Autodesk Inventor part; units mm, degrees
ref_plane "YZ Plane" through (0, 0, 0) normal (1, 0, 0) x (0, 1, 0)
ref_plane "XZ Plane" through (0, 0, 0) normal (0, 1, 0) x (-1, 0, 0)
ref_plane "XY Plane" through (0, 0, 0) normal (0, 0, 1) x (1, 0, 0)
sketch "Sketch1" plane through (0, 0, 0) normal (0, 0, 1) x (1, 0, 0)
  line L0 (-15.875, -28.575) -> (25.4, -28.575)
  line L1 (25.4, 28.575) -> (-15.875, 28.575)
  line L2 (-28.575, 15.875) -> (-28.575, -15.875)
  line L3 (-28.575, -28.575) -> (28.575, 28.575) construction
  line L4 (28.575, -28.575) -> (-28.575, 28.575) construction
  arc A0 (-15.875, 28.575) -> (-28.575, 15.875) centre (-15.875, 15.875) ccw
  arc A1 (-28.575, -15.875) -> (-15.875, -28.575) centre (-15.875, -15.875) ccw
  arc A2 (28.575, 25.4) -> (25.4, 28.575) centre (25.4, 25.4) ccw
  arc A3 (25.4, -28.575) -> (28.575, -25.4) centre (25.4, -25.4) ccw
  arc A4 (17.9256, 1.27) -> (17.9256, -1.27) centre (0, 0) ccw
  line L5 (18.2118, 5.08) -> (18.2118, -5.08) construction
  line L6 (17.9256, 1.27) -> (28.575, 1.27)
  line L7 (17.9256, -1.27) -> (28.575, -1.27)
  line L8 (28.575, -25.4) -> (28.575, -1.27)
  line L9 (28.575, 1.27) -> (28.575, 25.4)
  point P0 (23.2503, 1.27)
  point P1 (23.2503, -1.27)
  dimension "d0" = 57.15
  dimension "d1" = 57.15
  dimension "d2" = 12.7
  dimension "d3" = 3.175
  dimension "d5" = 10.16
  dimension "d8" = 28.575
  dimension "d11" = 57.15
  dimension "d14" = 2.54
  dimension "d23" = 35.941
extrude "Extrusion1" add sketch "Sketch1" along normal blind 17.78
sketch "Sketch2" plane through (17.9256, -1.27, 0) normal (0, 1, 0) x (1, 0, 0)
  line L0 (0, 0) -> (10.6494, 0)
  line L1 (0, 0) -> (0, -17.78)
  line L2 (10.6494, -17.78) -> (0, -17.78)
  line L3 (10.6494, 0) -> (10.6494, -17.78)
  circle A0 centre (5.2706, -8.89) radius 1.27
  point P0 (-17.9256, 0)
  dimension "d15" = 2.54
hole "Hole1" at (23.1962, -1.27, 8.89) direction (0, -1, 0) diameter 2.54 end through all
sketch "Sketch3" plane through (-15.875, -28.575, 0) normal (0, -1, 0) x (1, 0, 0)
  circle A0 centre (39.0712, 8.89) radius 1.27
  point P0 (15.875, 0)
  point P1 (38.1, 9.7084)
  point P2 (38.1, 8.0716)
hole "Hole2" at (23.1962, -28.575, 8.89) direction (0, 1, 0) diameter 4.064 end through all counterbore diameter 7.62 counterbore depth 6.35
sketch "Sketch4" plane through (0, 0, 17.78) normal (0, 0, 1) x (1, 0, 0)
  point P0 (0, 0)
sketch "Sketch5" plane through (0, 0, 17.78) normal (0, 0, 1) x (1, 0, 0)
  point P0 (0, 0)
sketch "Sketch6" plane through (0, 0, 17.78) normal (0, 0, 1) x (1, 0, 0)
  line L0 (25.4, 28.575) -> (-15.875, 28.575)
  arc A0 (-15.875, 28.575) -> (-28.575, 15.875) centre (-15.875, 15.875) ccw
  line L1 (-28.575, 15.875) -> (-28.575, -15.875)
  arc A1 (-28.575, -15.875) -> (-15.875, -28.575) centre (-15.875, -15.875) ccw
  line L2 (-15.875, -28.575) -> (25.4, -28.575)
  arc A2 (25.4, -28.575) -> (28.575, -25.4) centre (25.4, -25.4) ccw
  line L3 (28.575, -25.4) -> (28.575, -1.27)
  line L4 (28.575, -1.27) -> (17.9256, -1.27)
  arc A3 (17.9256, 1.27) -> (17.9256, -1.27) centre (0, 0) ccw
  line L5 (17.9256, 1.27) -> (28.575, 1.27)
  line L6 (28.575, 1.27) -> (28.575, 25.4)
  arc A4 (28.575, 25.4) -> (25.4, 28.575) centre (25.4, 25.4) ccw
  circle A5 centre (-19.685, -19.685) radius 1.27
  circle A6 centre (-19.685, 19.685) radius 1.27
  dimension "d31" = 2.54
  dimension "d32" = 3.81
  dimension "d33" = 3.81
  dimension "d34" = 2.54
  dimension "d35" = 3.81
  dimension "d36" = 3.81
extrude "Extrusion2" cut sketch "Sketch6" against normal blind 25.4 contours A5 | A6
properties part number "mOTORHOLDER"
Here's how the part is built. I have some questions about the finished solid (model axes, mm). A direction names the side the tool comes from. Give positions to 0.01 mm unless a question says otherwise; leave off trailing zeros. Order: outer loops, then holes, each group sorted by start corner. A loop starts at its lowest first (then second) coordinate and runs counter-clockwise, first axis right, second up. Notation, with made-up numbers: (12.25, 66.5) -> (29.25, 66.5) arc R6 cw to (29.25, 77.5) -> close; hole circle Ø8 at (32.5, 9.5). An arc over 180 degrees is marked (long way). Use a Markdown table: item, result. Add a question column.
Item 1: For faces 1 (the face through (24.4, -1.27, 6.8)), 2 (the face through (24.655, -25.356, 5.371)), 3 (the face through (-28.575, 0, 9)), which set-ups out of +Z, -Z, +X, -X, +Y, -Y let a thin tool reach every point of the face, with its end or its side?
Item 2: I need wall thicknesses on line 1 (X direction, y = 12, z = 8.75) (3 decimals); line 2 (Y direction, x = 0, z = 10.25) (3 decimals); line 3 (X direction, y = -11, z = 9.75) (3 decimals). Which ranges of each line are inside material? Lowest first, please.
Item 3: Imagine slicing it at A-A on z = 8.89. Please give me the cut outline in (x, y) (3 decimals), plus the area to 3 significant figures.
Item 4: Imagine slicing it at D-D on y = 24.5. Please give me the cut outline in (x, z) (3 decimals).
Item 5: Will this pin go through, and if not, where does the flat tip stop? pin 1 (3.5 mm diameter, centred on x = 23.2, z = 8.89, fed in from -Y) (1 decimal).
Item 6: Imagine slicing it at C-C on x = 0. Please give me the cut outline in (y, z) (3 decimals), plus the area to 3 significant figures.
Item 7: Imagine slicing it at B-B on y = -7.5. Please give me the cut outline in (x, z) (3 decimals), plus the area to 3 significant figures.
Item 8: If we mould it in two halves opening along Z, with no side actions, what happens to faces 4 (the face through (24.999, 15.114, 7.952)), 5 (the face through (-13, 13, 0)), 6 (the face through (25, -22.225, 7)), 7 (the face through (27.62, 27.67, 8.77))? For each: pulls with the +Z half, pulls with the -Z half, needs draft (parallel to the pull), parting line crosses it, or undercut.
Data:
| question | item | result |
|---|---|---|
| 1 | face 1 | +Z, -Z, +X |
| 1 | face 2 | -Y |
| 1 | face 3 | +Z, -Z, -X, +Y, -Y |
| 2 | line 1 | x = -28.575 to -13.377, 13.377 to 21.169, 25.223 to 28.575 |
| 2 | line 2 | y = -28.575 to -17.971, 17.971 to 28.575 |
| 2 | line 3 | x = -28.575 to -14.211, 14.211 to 21.355, 25.037 to 28.575 |
| 3 | outline | (-28.575, -15.875) arc R12.7 ccw to (-15.875, -28.575) -> (19.386, -28.575) -> (19.386, -22.225) -> (21.164, -22.225) -> (21.164, -1.27) -> (17.926, -1.27) arc R17.971 cw (long way) to (17.926, 1.27) -> (21.164, 1.27) -> (21.164, 28.575) -> (-15.875, 28.575) arc R12.7 ccw to (-28.575, 15.875) -> close; (25.228, -22.225) -> (27.006, -22.225) -> (27.006, -28.139) arc R3.175 ccw to (28.575, -25.4) -> (28.575, -1.27) -> (25.228, -1.27) -> close; (25.228, 1.27) -> (28.575, 1.27) -> (28.575, 25.4) arc R3.175 ccw to (25.4, 28.575) -> (25.228, 28.575) -> close; hole circle Ø2.54 at (-19.685, -19.685); hole circle Ø2.54 at (-19.685, 19.685) |
| 3 | area | 1,900 mm² |
| 4 | outline | (-25.197, 0) -> (28.575, 0) -> (28.575, 17.78) -> (-25.197, 17.78) -> close; hole circle Ø4.064 at (23.196, 8.89) |
| 5 | pin 1 | passes through |
| 6 | outline | (-28.575, 0) -> (-17.971, 0) -> (-17.971, 17.78) -> (-28.575, 17.78) -> close; (17.971, 0) -> (28.575, 0) -> (28.575, 17.78) -> (17.971, 17.78) -> close |
| 6 | area | 377 mm² |
| 7 | outline | (-28.575, 0) -> (-16.331, 0) -> (-16.331, 17.78) -> (-28.575, 17.78) -> close; (16.331, 0) -> (28.575, 0) -> (28.575, 17.78) -> (16.331, 17.78) -> close; hole circle Ø4.064 at (23.196, 8.89) |
| 7 | area | 422 mm² |
| 8 | face 4 | undercut |
| 8 | face 5 | pulls with the -Z half |
| 8 | face 6 | undercut |
| 8 | face 7 | needs draft |
